Design review of the part built by this model. Coordinates are the model's own, in mm. A direction names the side the tool comes from. Round coordinates to 2 decimals unless told otherwise and drop trailing zeros. Order: outer loops, then holes, each group sorted by start corner. A loop starts at its lowest first (then second) coordinate and runs counter-clockwise, first axis right, second up. Notation, with made-up numbers: M 83,48.5 L 117,48.5 A25 ccw 117,64.5 Z; hole C 74,89 d11. An arc over 180 degrees is marked long. Write each question's results on one line, items separated by ' | '. Start each with the question number.
Item 1: Clearance check with flat-ended pins moving along their axes: pin 1 (1 mm diameter, centred on x = 2, z = -4.5, fed in from +Y); pin 2 (4 mm diameter, centred on y = -9.5, z = -4, fed in from +X); pin 3 (5 mm diameter, centred on y = 6, z = -5, fed in from -X); pin 4 (2 mm diameter, centred on x = 9.72, y = -0.16, fed in from +Z). State where each tip first meets the part, or that it passes through.
Item 2: The part is to be moulded in two halves that separate along Z. For faces 3 (the flat face through (3, 0, 3)), 4 (the flat face through (3, 10, 0)), 5 (the cylindrical face through (11.945, -0.286, 1.521)), 6 (the flat face through (-3, 10, -3)), say which applies: +Z half, -Z half, draft (parallel to the pull), parting line (faces both ways), or undercut.
Item 3: Take a section at A-A, the plane x = 0. Write out the cut boundary in (y, z) (3 decimals), plus the area to 3 significant figures.
Item 4: Wall thickness on line 1 (Z direction, x = 11.5, y = 5.75); line 2 (Y direction, x = 0, z = 1.25) (3 decimals); line 3 (Y direction, x = 9, z = 2.5): over which ranges is each line inside the solid? List them lowest first. Write a range as [from, to].
Item 5: Take a section at C-C, the plane z = -3.75. Write out the cut boundary in (x, y) (3 decimals), plus the area to 3 significant figures.
Item 6: Take a section at B-B, the plane y = -0.75. Write out the cut boundary in (x, z), plus the area to 3 significant figures.
Item 7: Take a section at D-D, the plane y = -10.5. Write out the cut boundary in (x, z).
Item 8: Machinability: for faces 1 (the flat face through (0, -2, 0)), 2 (the cylindrical face through (8.587, -0.105, -1.437)), which of the approach directions +Z, -Z, +X, -X, +Y, -Y give a long, thin tool a straight path to every point of the face, cutting with its end or side? Answer none if there is none.
```python
from build123d import *
from build123d.topology import SkipClean

# Parameters (mm, degrees)
SKETCH1_R               = 13
SKETCH1_R_2             = 10
SKETCH1_R_3             = 2.575
BOSS_EXTRUDE4_DEPTH     = 3
BOSS_EXTRUDE5_START     = 3
SKETCH5_R               = 10
BOSS_EXTRUDE5_DEPTH     = 3
BOSS_EXTRUDE6_OUTLINE_R = 13
BOSS_EXTRUDE6_DEPTH     = 3
SKETCH8_R               = 1.136174382
SKETCH8_R_2             = 2.601730121
CUT_EXTRUDE2_DEPTH      = 14


# Read off the part's stored shape, not the designer's step: Boss-Extrude6
with BuildPart() as part:
    # Sketch1 → Boss-Extrude4 (new body)
    # profile 1 of 2: a face of its own
    with BuildSketch(Plane.XY):
        Circle(SKETCH1_R)
        Circle(SKETCH1_R_2, mode=Mode.SUBTRACT)
    # profile 2 of 2: a face of its own
    with BuildSketch(Plane.XY):
        Circle(SKETCH1_R_2)
        Circle(SKETCH1_R_3, mode=Mode.SUBTRACT)
    extrude(amount=BOSS_EXTRUDE4_DEPTH)

    # Sketch5 → Boss-Extrude5 (add)
    with SkipClean():  # the faces are left unmerged after this step: merging them gives an invalid solid
        with BuildSketch(Plane(origin=(0, 0, 0), x_dir=(-1, 0, 0), z_dir=(0, 0, -1)).offset(BOSS_EXTRUDE5_START)):
            Circle(SKETCH5_R)
            with BuildLine():
                Line((2.056240501, 1.55), (-2.056240501, 1.55))
                ThreePointArc((-2.056240501, 1.55), (-2.575, 0), (-2.056240501, -1.55))
                Line((-2.056240501, -1.55), (2.056240501, -1.55))
                ThreePointArc((2.056240501, -1.55), (2.575, 0), (2.056240501, 1.55))
            make_face(mode=Mode.SUBTRACT)
        extrude(amount=-BOSS_EXTRUDE5_DEPTH)

    # Boss-Extrude6 outline → Boss-Extrude6 (add)
    with SkipClean():  # the faces are left unmerged after this step: merging them gives an invalid solid
        with BuildSketch(Plane(origin=(0, 0, -3), x_dir=(-1, 0, 0), z_dir=(0, 0, -1))):
            Circle(BOSS_EXTRUDE6_OUTLINE_R)
            with BuildLine():
                Line((-2.056240501, 1.55), (2.056240501, 1.55))
                ThreePointArc((2.056240501, 1.55), (2.575, 0), (2.056240501, -1.55))
                Line((2.056240501, -1.55), (-2.056240501, -1.55))
                ThreePointArc((-2.056240501, -1.55), (-2.575, 0), (-2.056240501, 1.55))
            make_face(mode=Mode.SUBTRACT)
        extrude(amount=BOSS_EXTRUDE6_DEPTH)

    # Sketch8 → Cut-Extrude2 (cut)
    with SkipClean():  # the faces are left unmerged after this step: merging them gives an invalid solid
        with BuildSketch(Plane.XY.offset(3)):
            with Locations((9.721913819, -0.155301554)):
                Circle(SKETCH8_R)
            with Locations((14.544737257, -0.386006821)):
                Circle(SKETCH8_R_2)
        extrude(amount=-CUT_EXTRUDE2_DEPTH, mode=Mode.SUBTRACT)


solid = part.part
```
Results list:
1) pin 1: y = 12.91 | pin 2: x = 10.62 | pin 3: x = -12.52 | pin 4: through
2) face 3: +Z half | face 4: undercut | face 5: draft | face 6: undercut
3) outline: M -13,-6 L -1.55,-6 L -1.55,0 L -2.575,0 L -2.575,3 L -13,3 L -13,0 L -10,0 L -10,-3 L -13,-3 Z; M 1.55,-6 L 13,-6 L 13,-3 L 10,-3 L 10,0 L 13,0 L 13,3 L 2.575,3 L 2.575,0 L 1.55,0 Z | area: 182 mm²
4) line 1: [-6, -3], [0, 3] | line 2: [-13, -2.575], [2.575, 13] | line 3: [-9.38, -1.03], [0.72, 9.38]
5) outline: M 12.793,-2.31 A2.602 cw 12.898,1.628 A13 ccw long Z; hole M -2.056,-1.55 L 2.056,-1.55 A2.575 ccw 2.056,1.55 L -2.056,1.55 A2.575 ccw Z; hole C 9.722,-0.155 d2.272 | area: 509 mm²
6) outline: M -12.98,-6 L -2.46,-6 L -2.46,3 L -12.98,3 L -12.98,0 L -9.97,0 L -9.97,-3 L -12.98,-3 Z; M 2.46,-6 L 8.75,-6 L 8.75,3 L 2.46,3 Z; M 10.69,-6 L 11.97,-6 L 11.97,-3 L 10.69,-3 Z; M 10.69,0 L 11.97,0 L 11.97,3 L 10.69,3 Z | area: 150 mm²
7) outline: M -7.66,-6 L 7.66,-6 L 7.66,-3 L -7.66,-3 Z; M -7.66,0 L 7.66,0 L 7.66,3 L -7.66,3 Z
8) face 1: +Z | face 2: +Z, -Z
